from build123d import *

# Parameters (mm, degrees)
F0_R      = 2.54
F1_DEPTH  = 76.2
F3_DEPTH  = 5.588
F4_R      = 3.81
F5_DEPTH  = 2.54
F6_R      = 2.794
F7_DEPTH  = 2.54
F9_DEPTH  = 1.778
F11_R     = 2.54
F12_DEPTH = 1.27
F12_TAPER = -40
F13_R     = 0.127
F14_R     = 3.175
F15_DEPTH = 12.7
F16_R     = 2.921
F17_DEPTH = 5.08


with BuildPart() as f1:
    # F0 (on Top) → F1 (new body)
    with BuildSketch(Plane.XY):
        Circle(F0_R)
    extrude(amount=F1_DEPTH)

    # F2 (on Top) → F3 (join)
    with BuildSketch(Plane.XY):
        Polygon((2.2225, -3.8494829198), (4.445, 0), (2.2225, 3.8494829198), (-2.2225, 3.8494829198), (-4.445, 0), (-2.2225, -3.8494829198), align=None)
    extrude(amount=-F3_DEPTH)

    # F4 (on face) → F5 (join)
    with BuildSketch(Plane(origin=(0, 0, -5.588), x_dir=(1, 0, 0), z_dir=(0, 0, -1))):
        Circle(F4_R)
    extrude(amount=F5_DEPTH)

    # F6 (on face) → F7 (join)
    with BuildSketch(Plane(origin=(0, 0, -8.128), x_dir=(1, 0, 0), z_dir=(0, 0, -1))):
        Circle(F6_R)
    extrude(amount=F7_DEPTH)

    # F8 (on face) → F9 (join)
    with BuildSketch(Plane(origin=(0, 0, -10.668), x_dir=(1, 0, 0), z_dir=(0, 0, -1))):
        Polygon((-3.5949849635, 3.3503722934), (-4.699, -1.4381621579), (-1.1040150365, -4.7885344513), (3.5949849635, -3.3503722934), (4.699, 1.4381621579), (1.1040150365, 4.7885344513), align=None)
    extrude(amount=F9_DEPTH)



with BuildPart() as f12:
    # F11 (on offset) → F12 (new body)
    with BuildSketch(Plane.XY.offset(1.27)):
        Circle(F11_R)
    extrude(amount=F12_DEPTH, taper=F12_TAPER)

    # F13
    f13_edges = [f12.edges().sort_by_distance(p)[0] for p in [
        (-3.605657, 0, 2.54),
    ]]
    fillet(f13_edges, radius=F13_R)


with BuildPart() as f1_1:
    add(f1.part)

    add(f12.part)  # F15 merges F12
    # F14 (on face) → F15 (join)
    with BuildSketch(Plane.XY.offset(2.54)):
        Circle(F14_R)
    extrude(amount=F15_DEPTH)

    # F16 (on face) → F17 (join)
    with BuildSketch(Plane.XY.offset(15.24)):
        Circle(F16_R)
    extrude(amount=F17_DEPTH)


solid = f1_1.part
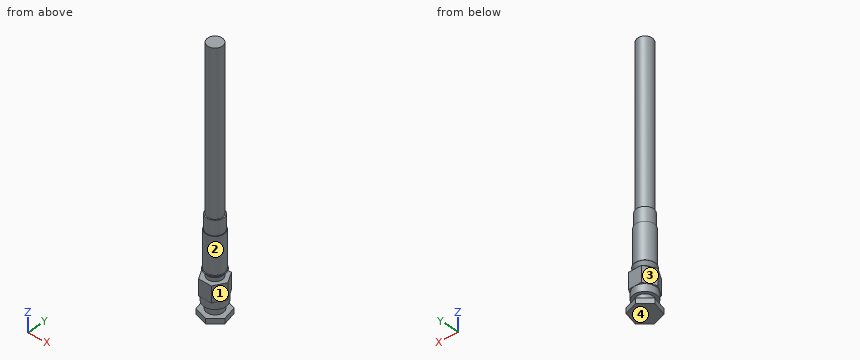
Part model, mm, in its own coordinate system. Face numbers are marked on the shaded views. A direction names the side the tool comes from. Coordinates: 2 decimals unless noted, no trailing zeros. Loops run counter-clockwise (first coordinate to the right, second up) from the corner with the lowest first, then second, coordinate; pieces in that order, holes last. Notation, with made-up numbers: M -22,68 L 23,68 A23 cw 23,106 Z; hole C -4,2 d11. An arc over 180 degrees is marked long. Use a Markdown table: item, result. Add a question column.
Q1. Cut at A-A (z = 66.5). Write the cut outline in (x, y), and give its area (3 significant figures).
Q2. Pin check, flat tips, straight feed: P1, Ø1, axis at x = -2, y = 3.5, coming from the +Z side; P2, Ø1.3, axis at x = 0, z = -3.5, coming from the -Y side; P3, Ø2, axis at y = -2, z = 24.5, coming from the -X side. Stop position of each tip, or through.
Q3. Probe L1, parallel to Z at x = -1, y = -3.5; L2, parallel to Z at x = 3, y = -0.75; L3, parallel to Z at x = -1.25, y = 3. List the from-to ranges inside material, lowest first.
Q4. Which spindle directions (+Z, -Z, +X, -X, +Y, -Y) get a long thin tool onto all of the face, cutting with end or side? Do the marked faces 1, 2, 3 and 4. Say none if no direction does.
Worked out:
| question | item | result |
|---|---|---|
| 1 | outline | C 0,0 d5.08 |
| 1 | area | 20.3 mm2 |
| 2 | P1 | stops at z = 0 |
| 2 | P2 | stops at y = -3.85 |
| 2 | P3 | stops at x = -2.33 |
| 3 | L1 | z = -12.45 to -10.67, -8.13 to 0 |
| 3 | L2 | z = -12.45 to -10.67, -8.13 to 0, 1.93 to 15.24 |
| 3 | L3 | z = -12.45 to -10.67, -8.13 to 0, 2.12 to 2.54 |
| 4 | face 1 | +Z, +X, -Y |
| 4 | face 2 | +Z |
| 4 | face 3 | +Z, -X, +Y |
| 4 | face 4 | -Z, +X, -X, +Y, -Y |
